Here's the drawing with two shaded views (mm, measured from the low corner). I have some questions. A direction names the side the tool comes from. Coordinates: 2 decimals unless noted, no trailing zeros. Write each loop counter-clockwise with the first axis right and the second up, starting at its lowest first coordinate (ties: lowest second). Pieces come first, ordered by that corner, then holes.
Item 1: We'd pull the mould along Y, two halves only. Please class the marked faces 5, 6 and 7: +Y half, -Y half, draft (parallel to the pull), parting line (faces both ways), or undercut.
Item 2: I'm going to push flat-ended pins straight in: pin 1 Ø11.5 at (x, z) = (15, 14.5) entering from -Y; pin 2 Ø10 at (x, y) = (18.5, 39) entering from -Z; pin 3 Ø5.5 at (x, y) = (24.5, 5.5) entering from +Z. Where does each tip first touch, or does it pass through?
Item 3: If we section it at A-A (x = 34.5): Please give me the cut outline in (y, z), then the cut area to 3 significant figures.
Item 4: If we section it at B-B (z = 34): Please give me the cut outline in (x, y).
Item 5: If we section it at C-C (x = 15.5): Please give me the cut outline in (y, z), then the cut area to 3 significant figures.
Item 6: If I drill on line 1 (Z direction, x = 17, y = 41.5); line 2 (X direction, y = 57.5, z = 87); line 3 (Y direction, x = 12, z = 127), over which ranges is the centre line in solid material (lowest first)?
Item 7: For the marked faces 1, 2, 3 and 4, which set-ups out of +Z, -Z, +X, -X, +Y, -Y let a thin tool reach every point of the face, with its end or its side?
Item 8: If we section it at D-D (y = 73.5): Please give me the cut outline in (x, z), then the cut area to 3 significant figures.
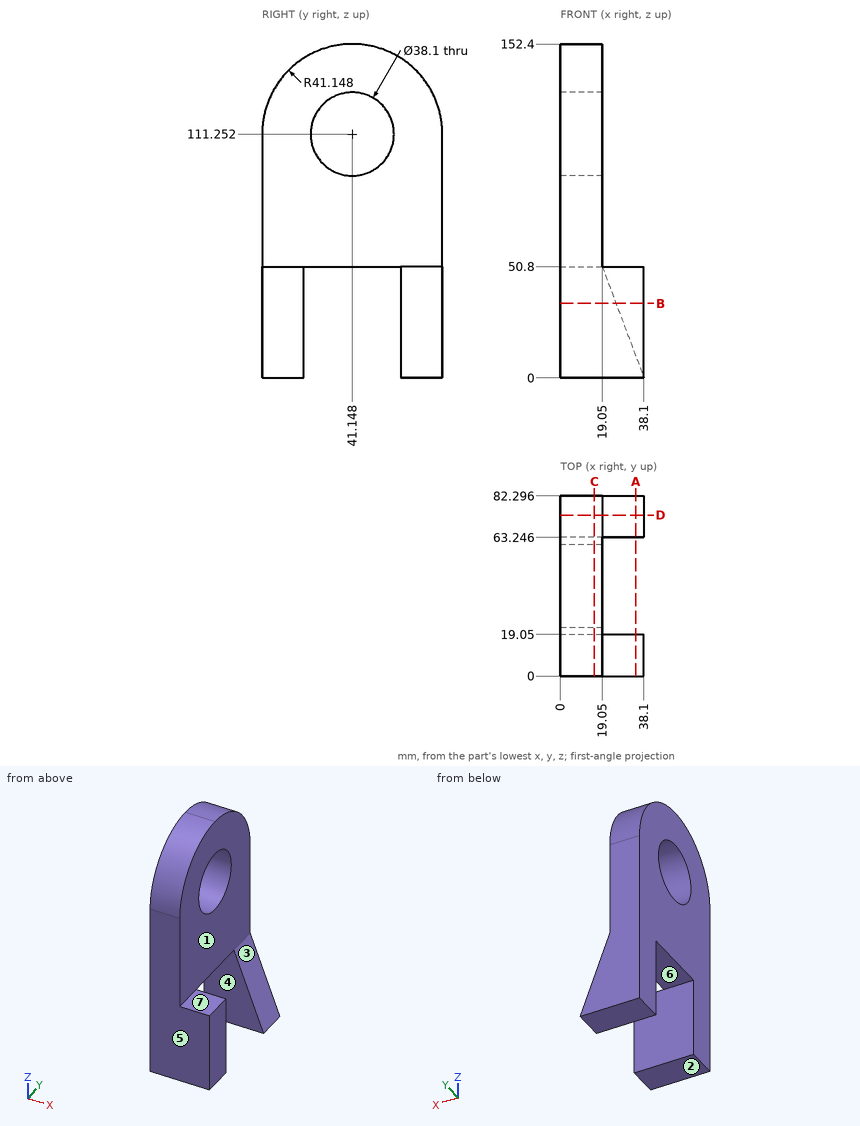
Answer list:
1. face 5: -Y half
1. face 6: undercut
1. face 7: draft
2. pin 1: stops at y = 0
2. pin 2: stops at z = 50.8
2. pin 3: stops at z = 50.8
3. outline: (0, 0) - (19.05, 0) - (19.05, 50.8) - (0, 50.8) - close; (63.25, 0) - (82.3, 0) - (82.3, 9.6) - (63.25, 9.6) - close
3. area: 1,150 mm2
4. outline: (0, 0) - (38.1, 0) - (38.1, 19.05) - (0, 19.05) - close; (0, 63.25) - (25.35, 63.25) - (25.35, 82.3) - (0, 82.3) - close
5. outline: (0, 0) - (19.05, 0) - (19.05, 50.8) - (63.25, 50.8) - (63.25, 0) - (82.3, 0) - (82.3, 111.25) arc R41.15 ccw to (41.15, 152.4) arc R41.15 ccw to (0, 111.25) - close; hole circle Ø38.1 at (41.15, 111.25)
5. area: 8,430 mm2
6. line 1: z = 50.8 to 92.21, 130.3 to 152.4
6. line 2: x = 0 to 19.05
6. line 3: y = 3.13 to 30.43, 51.87 to 79.16
7. face 1: +Z, +X, +Y, -Y
7. face 2: -Z, +X, -X, +Y, -Y
7. face 3: +Z, +X, +Y
7. face 4: -Z, +X, -X
8. outline: (0, 0) - (38.1, 0) - (19.05, 50.8) - (19.05, 136.68) - (0, 136.68) - close
8. area: 3,090 mm2
